Read the model definition and answer for the solid it produces. Units are mm, in the model's axes. A direction names the side the tool comes from. Give positions to 0.01 mm unless a question says otherwise; leave off trailing zeros. Order: outer loops, then holes, each group sorted by start corner. A loop starts at its lowest first (then second) coordinate and runs counter-clockwise, first axis right, second up. Notation, with made-up numbers: (54.5, 28.25) -> (112.5, 28.25) arc R17 ccw to (112.5, 37.25) -> close; hole circle Ø7 at (35.5, 68). An arc over 180 degrees is marked (long way). Use one line per item in the form item = value.
```python
from build123d import *

# Parameters (mm, degrees)
F1_DEPTH = 13
F2_R     = 2.1
F3_DEPTH = 13.001
F5_DEPTH = 5
F6_R     = 1


with BuildPart() as f1:
    # F0 (on Top) → F1 (new body)
    with BuildSketch(Plane.XY):
        with BuildLine():
            ThreePointArc((21.421995, -1.829787), (0, -21.5), (-21.421995, -1.829787))
            ThreePointArc((-21.421995, -1.829787), (-22.062043, -0.526836), (-23.414739, 0))
            Line((-23.414739, 0), (-36.445164, 0))
            ThreePointArc((-36.445164, 0), (-37.897607, -0.625078), (-38.44216, -2.109589))
            ThreePointArc((-38.44216, -2.109589), (0, -38.5), (38.44216, -2.109589))
            ThreePointArc((38.44216, -2.109589), (37.897607, -0.625078), (36.445164, 0))
            Line((36.445164, 0), (23.414739, 0))
            ThreePointArc((23.414739, 0), (22.062043, -0.526836), (21.421995, -1.829787))
        make_face()
    extrude(amount=F1_DEPTH)

    # F2 (on face) → F3 (cut, through all)
    with BuildSketch(Plane.XY):
        with Locations((-25.980762, -15)):
            Circle(F2_R)
        with Locations((0, -30)):
            Circle(F2_R)
        with Locations((25.980762, -15)):
            Circle(F2_R)
    extrude(amount=F3_DEPTH, mode=Mode.SUBTRACT)

    # F4 (on face) → F5 (cut)
    with BuildSketch(Plane.XY.offset(13)):
        Polygon((-23.815699, -18.75), (-21.650635, -15), (-23.815699, -11.25), (-28.145826, -11.25), (-30.310889, -15), (-28.145826, -18.75), align=None)
        Polygon((-2.165064, -33.75), (2.165064, -33.75), (4.330127, -30), (2.165064, -26.25), (-2.165064, -26.25), (-4.330127, -30), align=None)
        Polygon((23.815699, -18.75), (28.145826, -18.75), (30.310889, -15), (28.145826, -11.25), (23.815699, -11.25), (21.650635, -15), align=None)
    extrude(amount=-F5_DEPTH, mode=Mode.SUBTRACT)

    # F6
    f6_edges = [f1.edges().sort_by_distance(p)[0] for p in [
        (0, -21.5, 13),
        (22.062043, -0.526836, 13),
        (-22.062043, -0.526836, 13),
        (29.929952, 0, 13),
        (-29.929952, 0, 13),
        (37.897607, -0.625078, 13),
        (-37.897607, -0.625078, 13),
        (0, -38.5, 13),
        (-3.247595, -31.875, 13),
        (0, -33.75, 13),
        (3.247595, -31.875, 13),
        (3.247595, -28.125, 13),
        (0, -26.25, 13),
        (-3.247595, -28.125, 13),
        (-22.733167, -16.875, 13),
        (-22.733167, -13.125, 13),
        (-25.980762, -11.25, 13),
        (-29.228357, -13.125, 13),
        (-29.228357, -16.875, 13),
        (-25.980762, -18.75, 13),
        (22.733167, -16.875, 13),
        (25.980762, -18.75, 13),
        (29.228357, -16.875, 13),
        (29.228357, -13.125, 13),
        (25.980762, -11.25, 13),
        (22.733167, -13.125, 13),
    ]]
    fillet(f6_edges, radius=F6_R)


solid = f1.part
```
Item 1: Which of the six approach directions +Z, -Z, +X, -X, +Y, -Y give full straight-line access (tool end or side, diameter ignored) to faces 1 (the flat face through (0, -33.75, 10)), 2 (the cylindrical face through (-0.82, -38.49, 5.92)), 3 (the cylindrical face through (22.08, -0.51, 5.92))?
Checks:
face_1 = +Z
face_2 = +Z, -Z, -Y
face_3 = +Z, -Z, +Y
Item 2: Given pin 1 Ø2 at (x, y) = (-24, -14.5) entering from +Z; pin 2 Ø6 at (x, z) = (3, 11) entering from +Y; pin 3 Ø4.5 at (x, z) = (-25, 10) entering from -Y; pin 4 Ø2 at (x, z) = (0.5, 10.5) entering from -Y, each flat-ended and moving along its own axis, determine where each tip first touches the part or whether it passes through.
Checks:
pin_1 = 8
pin_2 = -20.65
pin_3 = -31.06
pin_4 = -38.5
Item 3: Determine the mould class of faces 4 (the flat face through (3.232, -31.901, 10.028)), 5 (the cylindrical face through (-37.882, -0.609, 5.916)), 6 (the cylindrical face through (37.91, -0.64, 5.92)), 7 (the cylindrical face through (22.454, -13.008, 12.715)) for opening direction X: +X half, -X half, draft (parallel to the pull), parting line (faces both ways), or undercut.
Checks:
face_4 = undercut
face_5 = -X half
face_6 = +X half
face_7 = undercut
Item 4: Straight lines are drawn through the part: L1, parallel to X at y = -15, z = 10.75; L2, parallel to X at y = -16, z = 11; L3, parallel to Y at x = -1.5, z = 5.5. For each, find the intervals that lie inside material, in ascending order. Write a range as from..to.
Checks:
L1 = -35.46..-30.31, -21.65..-15.4, 15.4..21.65, 30.31..35.46
L2 = -35.02..-29.73, -22.23..-14.36, 14.36..22.23, 29.73..35.02
L3 = -38.47..-31.47, -28.53..-21.45
Item 5: The part is cut by section B-B on z = 2.5. Give the vertices of the cut face in (x, y).
Checks:
outline = (-38.44, -2.11) arc R38.5 ccw to (38.44, -2.11) arc R2 ccw to (36.45, 0) -> (23.41, 0) arc R2 ccw to (21.42, -1.83) arc R21.5 cw to (-21.42, -1.83) arc R2 ccw to (-23.41, 0) -> (-36.45, 0) arc R2 ccw to start; hole circle Ø4.2 at (-25.98, -15); hole circle Ø4.2 at (0, -30); hole circle Ø4.2 at (25.98, -15)
Item 6: The part is cut by section A-A on x = 0. Give the vertices of the cut face in (y, z), and give its area (3 significant figures).
Checks:
outline = (-38.5, 0) -> (-32.1, 0) -> (-32.1, 8) -> (-33.75, 8) -> (-33.75, 12) arc R1 ccw to (-34.75, 13) -> (-37.5, 13) arc R1 ccw to (-38.5, 12) -> close; (-27.9, 0) -> (-21.5, 0) -> (-21.5, 12) arc R1 ccw to (-22.5, 13) -> (-25.25, 13) arc R1 ccw to (-26.25, 12) -> (-26.25, 8) -> (-27.9, 8) -> close
area = 149 mm²
